```python
from build123d import *

# Parameters (mm, degrees)
BLOCK_DEPTH                     = 29
TAP_DRILL_FOR_M8X1_0_TAP1_D     = 6
TAP_DRILL_FOR_M8X1_0_TAP1_DEPTH = 12.5
TAP_DRILL_FOR_M8X1_0_TAP1_TIP   = 1.561701152
F_6_0_6_DIAMETER_HOLE1_D        = 6


with BuildPart() as part:
    # Sketch2 → Block (new body, symmetric)
    with BuildSketch(Plane.XY):
        with BuildLine():
            Line((22, 0), (23.5, 1.5))
            Line((23.5, 1.5), (23.5, 17.499972901))
            Line((23.5, 17.499972901), (24, 17.999972901))
            Line((24, 17.999972901), (24, 32.999972901))
            Line((24, 32.999972901), (22.5, 34.5))
            Line((22.5, 34.5), (13.5, 34.5))
            Line((13.5, 34.5), (13.000005928, 34))
            Line((13.000005928, 34), (5.000005928, 34))
            Line((5.000005928, 34), (4.500011856, 34.5))
            Line((4.500011856, 34.5), (-4.499988144, 34.5))
            Line((-4.499988144, 34.5), (-4.999982216, 34))
            Line((-4.999982216, 34), (-12.999982216, 34))
            Line((-12.999982216, 34), (-13.499976288, 34.5))
            Line((-13.499976288, 34.5), (-22.499976288, 34.5))
            Line((-22.499976288, 34.5), (-24, 32.999996612))
            Line((-24, 32.999996612), (-24, 26.499996612))
            Line((-24, 26.499996612), (-23.5, 25.999996612))
            Line((-23.5, 25.999996612), (-23.5, 1.5))
            Line((-23.5, 1.5), (-22, 0))
            Line((-22, 0), (-11.5, 0))
            Line((-11.5, 0), (-11.5, 0.6))
            Line((-11.5, 0.6), (-7.7, 4.393650985))
            Line((-7.7, 4.393650985), (-7.7, 7.773650985))
            Line((-7.7, 7.773650985), (-8.93, 9.0057095))
            ThreePointArc((-8.93, 9.0057095), (-9.805517545, 10.387881926), (-11.186224007, 11.2657095))
            Line((-11.186224007, 11.2657095), (-11.39587314, 11.4757095))
            Line((-11.39587314, 11.4757095), (-11.39587314, 13.5057095))
            Line((-11.39587314, 13.5057095), (-11.186224007, 13.7157095))
            ThreePointArc((-11.186224007, 13.7157095), (-9.805517545, 14.593537075), (-8.93, 15.9757095))
            Line((-8.93, 15.9757095), (-8.520685025, 16.3857095))
            Line((-8.520685025, 16.3857095), (8.520685025, 16.3857095))
            Line((8.520685025, 16.3857095), (8.93, 15.9757095))
            ThreePointArc((8.93, 15.9757095), (9.805517545, 14.593537075), (11.186224007, 13.7157095))
            Line((11.186224007, 13.7157095), (11.39587314, 13.5057095))
            Line((11.39587314, 13.5057095), (11.39587314, 11.4757095))
            Line((11.39587314, 11.4757095), (11.186224007, 11.2657095))
            ThreePointArc((11.186224007, 11.2657095), (9.805517545, 10.387881926), (8.93, 9.0057095))
            Line((8.93, 9.0057095), (7.7, 7.773650985))
            Line((7.7, 7.773650985), (7.7, 4.393650985))
            Line((7.7, 4.393650985), (11.5, 0.6))
            Line((11.5, 0.6), (11.5, 0))
            Line((11.5, 0), (22, 0))
        make_face()
    extrude(amount=BLOCK_DEPTH, both=True)

    # Tap Drill for M8x1.0 Tap1
    with Locations(Plane(origin=(0, 34.5, 0), x_dir=(1, 0, 0), z_dir=(0, 1, 0))):
        with Locations((17.5, 17.5), (-17.5, 17.5), (17.5, -17.5), (-17.5, -17.5)):
            Hole(TAP_DRILL_FOR_M8X1_0_TAP1_D / 2, depth=TAP_DRILL_FOR_M8X1_0_TAP1_DEPTH)
            with Locations((0, 0, -(TAP_DRILL_FOR_M8X1_0_TAP1_DEPTH + TAP_DRILL_FOR_M8X1_0_TAP1_TIP / 2))):  # 125° drill point
                Cone(0, TAP_DRILL_FOR_M8X1_0_TAP1_D / 2, TAP_DRILL_FOR_M8X1_0_TAP1_TIP, mode=Mode.SUBTRACT)

    # Ø6.0 (6) Diameter Hole1 (through all)
    with Locations(Plane(origin=(0, 0, -29), x_dir=(-1, 0, 0), z_dir=(0, 0, -1))):
        with Locations((0, 24.3857095)):
            Hole(F_6_0_6_DIAMETER_HOLE1_D / 2)


solid = part.part
```
Geometry check sheet. Reference: the model listing, model coordinates, mm. A direction names the side the tool comes from. Give positions to 0.01 mm unless a question says otherwise; leave off trailing zeros. Write each loop counter-clockwise with the first axis right and the second up, starting at its lowest first coordinate (ties: lowest second). Pieces come first, ordered by that corner, then holes. Notation, with made-up numbers: (8.5, -4.5) -> (48.5, -4.5) arc R37 cw to (48.5, 33.5) -> close; hole circle Ø10 at (-4, 34.25). An arc over 180 degrees is marked (long way). One line per question, with ' | ' between items.
Item 1: Scan lines: line 1 along Z through (x, y) = (-17.5, 29.75); line 2 along X through (y, z) = (29.75, 17.5); line 3 along X through (y, z) = (5, 14). Record each from-to range of solid material in increasing order.
Determined:
line 1: -29 to -20.5, -14.5 to 14.5, 20.5 to 29 | line 2: -24 to -20.5, -14.5 to 14.5, 20.5 to 24 | line 3: -23.5 to -7.7, 7.7 to 23.5
Item 2: Depth check by flat-ended pin: pin 1 (0.7 mm diameter, centred on y = 0, z = 0.5, fed in from +X); pin 2 (3.5 mm diameter, centred on x = 17.5, z = 17.5, fed in from +Y); pin 3 (3 mm diameter, centred on y = 6.5, z = 6.5, fed in from -X). Enter the tip coordinate at first touch or a pass-through.
Determined:
pin 1: x = 22.35 | pin 2: y = 21.35 | pin 3: x = -23.5
Item 3: Sectioned sample at B-B, the plane x = 2. Record the boundary of the cut face in (y, z).
Determined:
outline: (16.39, -29) -> (22.15, -29) -> (22.15, 29) -> (16.39, 29) -> close; (26.62, -29) -> (34.5, -29) -> (34.5, 29) -> (26.62, 29) -> close
Item 4: Draft check along X on faces 4 (the cylindrical face through (-9.79, 10.37, 0.41)), 5 (the flat face through (23.5, 9, 0)), 6 (the cylindrical face through (9.82, 10.4, 0.41)), 7 (the flat face through (0, 17, -29)). Enter one of: released by +X, released by -X, zero draft, split by the parting line, or undercut.
Determined:
face 4: undercut | face 5: released by +X | face 6: undercut | face 7: zero draft
Item 5: Sectioned sample at A-A, the plane y = 31. Record the boundary of the cut face in (x, z).
Determined:
outline: (-24, -29) -> (24, -29) -> (24, 29) -> (-24, 29) -> close; hole circle Ø6 at (-17.5, -17.5); hole circle Ø6 at (-17.5, 17.5); hole circle Ø6 at (17.5, -17.5); hole circle Ø6 at (17.5, 17.5)
Item 6: Access from +Z, -Z, +X, -X, +Y, -Y to the whole of each face (thin tool, end or side, straight path). Record for faces 1 (the flat face through (-23.5, 14, 0)), 2 (the cylindrical face through (9.8, 14.6, 0.4)), 3 (the flat face through (9.573, 2.523, 0.406)).
Determined:
face 1: +Z, -Z, -X, -Y | face 2: +Z, -Z | face 3: +Z, -Z, -Y
